Source: CAD feature listing. Evaluate the final solid. Frame: model axes, mm. Round coordinates to 2 decimals unless told otherwise and drop trailing zeros. Loops run counter-clockwise (first coordinate to the right, second up) from the corner with the lowest first, then second, coordinate; pieces in that order, holes last.
Item 1: Section query A-A on x = 211.5. Return loops of the section in (y, z) (3 decimals), then the cut area to 3 significant figures.
Item 2: First-contact query: P1, Ø4, axis at x = 88.9, z = -127, coming from the -Y side. Flat tip, straight axial feed; report the tip coordinate or a pass-through.
Item 3: Section query B-B on z = -200. Return loops of the section in (x, y) (3 decimals).
Item 4: Section query C-C on z = -260. Return loops of the section in (x, y) (3 decimals).
Item 5: Pull-direction query (Z, two-part tool) for faces 1 (the flat face through (227, 3.175, -261)), 2 (the flat face through (225, 0, -155)); classes: released by +Z, released by -Z, zero draft, split by the parting line, or undercut.
Item 6: Ray query, L1, parallel to X at y = 2.75, z = -76.2 (3 decimals); L2, parallel to X at y = 3.25, z = -118; L3, parallel to Z at x = 209, y = 4.5. Return the intervals inside material, ascending.
```python
from build123d import *

# Parameters (mm, degrees)
SKETCH1_W             = 457.2
SKETCH1_H             = 304.8
BOSS_EXTRUDE2_DEPTH   = 6.35
SKETCH1_5_OUTSIDE_W   = 569.104
SKETCH1_5_OUTSIDE_H   = 416.704
SKETCH1_5_OUTSIDE_W_2 = 457.2
SKETCH1_5_OUTSIDE_H_2 = 304.8
SKETCH1_5_OUTSIDE_R   = 3.175
CUT_EXTRUDE3_DEPTH    = 6.35
SKETCH5_W             = 241.3
SKETCH5_H             = 241.3
SKETCH5_W_2           = 203.2
SKETCH5_H_2           = 203.2
CUT_EXTRUDE7_DEPTH    = 3.175
SKETCH6_W             = 7.62
SKETCH6_H             = 31.75
CUT_EXTRUDE8_DEPTH    = 1.5875
SKETCH12_R            = 3.175
CUT_EXTRUDE13_DEPTH   = 6.35
FILLET1_R             = 6.35


with BuildPart() as part:
    # Sketch1 → Boss-Extrude2 (new body)
    with BuildSketch(Plane(origin=(0, 0, 0), x_dir=(1, 0, 0), z_dir=(0, 1, 0))):
        with Locations((228.314285714, 152.4)):
            Rectangle(SKETCH1_W, SKETCH1_H)
    extrude(amount=BOSS_EXTRUDE2_DEPTH)

    # Sketch1_5 outside → Cut-Extrude3 (cut)
    # profile 1 of 25: a face of its own
    with BuildSketch(Plane(origin=(0, 0, 0), x_dir=(1, 0, 0), z_dir=(0, 1, 0))):
        with Locations((228.314, 152.4)):
            Rectangle(SKETCH1_5_OUTSIDE_W, SKETCH1_5_OUTSIDE_H)
        with Locations((228.314285714, 152.4)):
            Rectangle(SKETCH1_5_OUTSIDE_W_2, SKETCH1_5_OUTSIDE_H_2, mode=Mode.SUBTRACT)
    # profile 2 of 25: a face of its own
    with BuildSketch(Plane(origin=(0, 0, 0), x_dir=(1, 0, 0), z_dir=(0, 1, 0))):
        with Locations(Location((38.1, 25.4, 0), (0, 0, 270))):
            Circle(SKETCH1_5_OUTSIDE_R)
    # profile 3 of 25: a face of its own
    with BuildSketch(Plane(origin=(0, 0, 0), x_dir=(1, 0, 0), z_dir=(0, 1, 0))):
        with Locations(Location((38.1, 76.2, 0), (0, 0, 270))):
            Circle(SKETCH1_5_OUTSIDE_R)
    # profile 4 of 25: a face of its own
    with BuildSketch(Plane(origin=(0, 0, 0), x_dir=(1, 0, 0), z_dir=(0, 1, 0))):
        with Locations(Location((38.1, 127, 0), (0, 0, 270))):
            Circle(SKETCH1_5_OUTSIDE_R)
    # profile 5 of 25: a face of its own
    with BuildSketch(Plane(origin=(0, 0, 0), x_dir=(1, 0, 0), z_dir=(0, 1, 0))):
        with Locations(Location((38.1, 228.6, 0), (0, 0, 270))):
            Circle(SKETCH1_5_OUTSIDE_R)
    # profile 6 of 25: a face of its own
    with BuildSketch(Plane(origin=(0, 0, 0), x_dir=(1, 0, 0), z_dir=(0, 1, 0))):
        with Locations(Location((38.1, 279.4, 0), (0, 0, 270))):
            Circle(SKETCH1_5_OUTSIDE_R)
    # profile 7 of 25: a face of its own
    with BuildSketch(Plane(origin=(0, 0, 0), x_dir=(1, 0, 0), z_dir=(0, 1, 0))):
        with Locations(Location((38.1, 177.8, 0), (0, 0, 270))):
            Circle(SKETCH1_5_OUTSIDE_R)
    # profile 8 of 25: a face of its own
    with BuildSketch(Plane(origin=(0, 0, 0), x_dir=(1, 0, 0), z_dir=(0, 1, 0))):
        with Locations(Location((88.9, 279.4, 0), (0, 0, 270))):
            Circle(SKETCH1_5_OUTSIDE_R)
    # profile 9 of 25: a face of its own
    with BuildSketch(Plane(origin=(0, 0, 0), x_dir=(1, 0, 0), z_dir=(0, 1, 0))):
        with Locations(Location((88.9, 228.6, 0), (0, 0, 270))):
            Circle(SKETCH1_5_OUTSIDE_R)
    # profile 10 of 25: a face of its own
    with BuildSketch(Plane(origin=(0, 0, 0), x_dir=(1, 0, 0), z_dir=(0, 1, 0))):
        with Locations(Location((88.9, 177.8, 0), (0, 0, 270))):
            Circle(SKETCH1_5_OUTSIDE_R)
    # profile 11 of 25: a face of its own
    with BuildSketch(Plane(origin=(0, 0, 0), x_dir=(1, 0, 0), z_dir=(0, 1, 0))):
        with Locations(Location((88.9, 127, 0), (0, 0, 270))):
            Circle(SKETCH1_5_OUTSIDE_R)
    # profile 12 of 25: a face of its own
    with BuildSketch(Plane(origin=(0, 0, 0), x_dir=(1, 0, 0), z_dir=(0, 1, 0))):
        with Locations(Location((88.9, 76.2, 0), (0, 0, 270))):
            Circle(SKETCH1_5_OUTSIDE_R)
    # profile 13 of 25: a face of its own
    with BuildSketch(Plane(origin=(0, 0, 0), x_dir=(1, 0, 0), z_dir=(0, 1, 0))):
        with Locations(Location((88.9, 25.4, 0), (0, 0, 270))):
            Circle(SKETCH1_5_OUTSIDE_R)
    # profile 14 of 25: a face of its own
    with BuildSketch(Plane(origin=(0, 0, 0), x_dir=(1, 0, 0), z_dir=(0, 1, 0))):
        with Locations(Location((368.3, 279.4, 0), (0, 0, 270))):
            Circle(SKETCH1_5_OUTSIDE_R)
    # profile 15 of 25: a face of its own
    with BuildSketch(Plane(origin=(0, 0, 0), x_dir=(1, 0, 0), z_dir=(0, 1, 0))):
        with Locations(Location((419.1, 228.6, 0), (0, 0, 270))):
            Circle(SKETCH1_5_OUTSIDE_R)
    # profile 16 of 25: a face of its own
    with BuildSketch(Plane(origin=(0, 0, 0), x_dir=(1, 0, 0), z_dir=(0, 1, 0))):
        with Locations(Location((419.1, 177.8, 0), (0, 0, 270))):
            Circle(SKETCH1_5_OUTSIDE_R)
    # profile 17 of 25: a face of its own
    with BuildSketch(Plane(origin=(0, 0, 0), x_dir=(1, 0, 0), z_dir=(0, 1, 0))):
        with Locations(Location((368.3, 127, 0), (0, 0, 270))):
            Circle(SKETCH1_5_OUTSIDE_R)
    # profile 18 of 25: a face of its own
    with BuildSketch(Plane(origin=(0, 0, 0), x_dir=(1, 0, 0), z_dir=(0, 1, 0))):
        with Locations(Location((368.3, 76.2, 0), (0, 0, 270))):
            Circle(SKETCH1_5_OUTSIDE_R)
    # profile 19 of 25: a face of its own
    with BuildSketch(Plane(origin=(0, 0, 0), x_dir=(1, 0, 0), z_dir=(0, 1, 0))):
        with Locations(Location((368.3, 25.4, 0), (0, 0, 270))):
            Circle(SKETCH1_5_OUTSIDE_R)
    # profile 20 of 25: a face of its own
    with BuildSketch(Plane(origin=(0, 0, 0), x_dir=(1, 0, 0), z_dir=(0, 1, 0))):
        with Locations(Location((419.1, 279.4, 0), (0, 0, 270))):
            Circle(SKETCH1_5_OUTSIDE_R)
    # profile 21 of 25: a face of its own
    with BuildSketch(Plane(origin=(0, 0, 0), x_dir=(1, 0, 0), z_dir=(0, 1, 0))):
        with Locations(Location((419.1, 127, 0), (0, 0, 270))):
            Circle(SKETCH1_5_OUTSIDE_R)
    # profile 22 of 25: a face of its own
    with BuildSketch(Plane(origin=(0, 0, 0), x_dir=(1, 0, 0), z_dir=(0, 1, 0))):
        with Locations(Location((419.1, 76.2, 0), (0, 0, 270))):
            Circle(SKETCH1_5_OUTSIDE_R)
    # profile 23 of 25: a face of its own
    with BuildSketch(Plane(origin=(0, 0, 0), x_dir=(1, 0, 0), z_dir=(0, 1, 0))):
        with Locations(Location((419.1, 25.4, 0), (0, 0, 270))):
            Circle(SKETCH1_5_OUTSIDE_R)
    # profile 24 of 25: a face of its own
    with BuildSketch(Plane(origin=(0, 0, 0), x_dir=(1, 0, 0), z_dir=(0, 1, 0))):
        with Locations(Location((368.3, 177.8, 0), (0, 0, 270))):
            Circle(SKETCH1_5_OUTSIDE_R)
    # profile 25 of 25: a face of its own
    with BuildSketch(Plane(origin=(0, 0, 0), x_dir=(1, 0, 0), z_dir=(0, 1, 0))):
        with Locations(Location((368.3, 228.6, 0), (0, 0, 270))):
            Circle(SKETCH1_5_OUTSIDE_R)
    extrude(amount=CUT_EXTRUDE3_DEPTH, mode=Mode.SUBTRACT)

    # Sketch5 → Cut-Extrude7 (cut)
    with BuildSketch(Plane(origin=(0, 6.35, 0), x_dir=(1, 0, 0), z_dir=(0, 1, 0))):
        with Locations((228.6, 152.4)):
            Rectangle(SKETCH5_W, SKETCH5_H)
        with Locations((228.6, 152.4)):
            Rectangle(SKETCH5_W_2, SKETCH5_H_2, mode=Mode.SUBTRACT)
    extrude(amount=-CUT_EXTRUDE7_DEPTH, mode=Mode.SUBTRACT)

    # Sketch6 → Cut-Extrude8 (cut)
    with BuildSketch(Plane(origin=(0, 6.35, 0), x_dir=(1, 0, 0), z_dir=(0, 1, 0))):
        with Locations((229.235, 15.875)):
            Rectangle(SKETCH6_W, SKETCH6_H)
    extrude(amount=-CUT_EXTRUDE8_DEPTH, mode=Mode.SUBTRACT)

    # Sketch12 → Cut-Extrude13 (cut)
    with BuildSketch(Plane.XZ):
        with Locations(Location((12.7, -25.4, 0), (0, 0, 270))):
            Circle(SKETCH12_R)
        with Locations(Location((12.7, -279.4, 0), (0, 0, 270))):
            Circle(SKETCH12_R)
        with Locations(Location((444.5, -25.4, 0), (0, 0, 270))):
            Circle(SKETCH12_R)
        with Locations(Location((444.5, -279.4, 0), (0, 0, 270))):
            Circle(SKETCH12_R)
    extrude(amount=-CUT_EXTRUDE13_DEPTH, mode=Mode.SUBTRACT)

    # Fillet1
    fillet1_edges = [part.edges().sort_by_distance(p)[0] for p in [
        (107.95, 4.7625, -273.05),
        (349.25, 4.7625, -273.05),
        (349.25, 4.7625, -31.75),
        (107.95, 4.7625, -31.75),
    ]]
    fillet(fillet1_edges, radius=FILLET1_R)


solid = part.part
```
Data:
1. outline: (0, -304.8) - (6.35, -304.8) - (6.35, -273.05) - (3.175, -273.05) - (3.175, -254) - (6.35, -254) - (6.35, -50.8) - (3.175, -50.8) - (3.175, -31.75) - (6.35, -31.75) - (6.35, 0) - (0, 0) - close
1. area: 1,810 mm2
2. P1: passes through
3. outline: (-0.286, 0) - (456.914, 0) - (456.914, 6.35) - (349.25, 6.35) - (349.25, 3.175) - (330.2, 3.175) - (330.2, 6.35) - (127, 6.35) - (127, 3.175) - (107.95, 3.175) - (107.95, 6.35) - (-0.286, 6.35) - close
4. outline: (-0.286, 0) - (456.914, 0) - (456.914, 6.35) - (349.25, 6.35) - (349.25, 3.175) - (107.95, 3.175) - (107.95, 6.35) - (-0.286, 6.35) - close
5. face 1: undercut
5. face 2: zero draft
6. L1: x = -0.286 to 34.925, 41.275 to 85.725, 92.075 to 365.125, 371.475 to 415.925, 422.275 to 456.914
6. L2: x = -0.29 to 107.95, 127 to 330.2, 349.25 to 456.91
6. L3: z = -304.8 to -273.05, -254 to -50.8, -31.75 to 0
